from build123d import *

# Parameters (mm, degrees)
F0_R     = 10.5
F0_R_2   = 7.5
F1_DEPTH = 1.55
F2_R     = 1.49999


# Not quite as in the source:
# - a fillet or chamfer is up to 0.001 mm smaller than in the source, because OpenCascade refuses the exact size


with BuildPart() as f1:
    # F0 (on Front) → F1 (new body, symmetric)
    with BuildSketch(Plane.XZ):
        Circle(F0_R)
        Circle(F0_R_2, mode=Mode.SUBTRACT)
    extrude(amount=F1_DEPTH, both=True)

    # F2 (radius 1.5 in the source; OpenCascade refuses exactly that, so slightly less here)
    f2_edges = [f1.edges().sort_by_distance(p)[0] for p in [
        (-10.5, -1.55, 0),
        (-10.5, 1.55, 0),
        (-7.5, 1.55, 0),
        (-7.5, -1.55, 0),
    ]]
    fillet(f2_edges, radius=F2_R)


solid = f1.part
Check sheet for the modelled part. Datum: model origin and axes. Units: mm. Give positions to 0.01 mm unless a question says otherwise; leave off trailing zeros. Write each loop counter-clockwise with the first axis right and the second up, starting at its lowest first coordinate (ties: lowest second). Pieces come first, ordered by that corner, then holes. Notation, with made-up numbers: (0, 86.25) -> (21, 86.25) arc R11 cw to (21, 92.25) -> close; hole circle Ø5 at (52.5, 84). An arc over 180 degrees is marked (long way). One line per item, written item: value. Start each with the question number.
Item 1: Gauge pin test, flat ends, axial feed: pin 1 (4 mm diameter, centred on x = -5.5, z = 2.5, fed in from +Y); pin 2 (1 mm diameter, centred on y = 1, z = 3.5, fed in from +X); pin 3 (6 mm diameter, centred on x = 2, z = 4.5, fed in from +Y). Record the tip position at first contact, or that the pin passes through.
Item 2: Section check D-D on y = 1.1. Record the cut outline in (x, z), then the cut area to 3 significant figures.
Item 3: Material ranges on probe 1 along Z at (x, y) = (0, 0); probe 2 along Z at (x, y) = (-3.5, 1.2); probe 3 along X at (y, z) = (-0.9, -6), recorded low to high. Write a range as from..to.
Item 4: Section check C-C on y = -1.25. Record the cut outline in (x, z).
Results list:
1. pin 1: y = 1.2
1. pin 2: x = 9.89
1. pin 3: y = 1.1
2. outline: circle Ø20.14 at (0, 0); hole circle Ø15.86 at (0, 0)
2. area: 121 mm²
3. probe 1: -10.5..-7.5, 7.5..10.5
3. probe 2: -9.33..-7.23, 7.23..9.33
3. probe 3: -8.29..-4.93, 4.93..8.29
4. outline: circle Ø19.8 at (0, 0); hole circle Ø16.2 at (0, 0)
